Geometry check sheet. Reference: the model listing, model coordinates, mm. A direction names the side the tool comes from. Coordinates: 2 decimals unless noted, no trailing zeros. Write each loop counter-clockwise with the first axis right and the second up, starting at its lowest first coordinate (ties: lowest second). Pieces come first, ordered by that corner, then holes. Notation, with made-up numbers: (57, -2) - (70, -2) arc R16 ccw to (70, 15) - close; hole circle Ø6 at (60, -15). An arc over 180 degrees is marked (long way). Answer as a JSON object with one key per item and string values. Group by question number.
from build123d import *

# Parameters (mm, degrees)
F1_DEPTH = 15
F2_W     = 3.3
F2_H     = 1
F2_W_2   = 6.2084717173
F3_DEPTH = 13.301
F4_R     = 5


with BuildPart() as f1:
    # F0 (on Top) → F1 (new body)
    with BuildSketch(Plane.XY):
        with BuildLine():
            Line((6.65, 0), (1.65, 0))
            ThreePointArc((1.65, 0), (0, -1.65), (-1.65, 0))
            Line((-1.65, 0), (-6.65, 0))
            ThreePointArc((-6.65, 0), (0, -6.65), (6.65, 0))
        make_face()
        with BuildLine():
            ThreePointArc((-1.65, 0), (0, 1.65), (1.65, 0))
            Line((1.65, 0), (6.65, 0))
            ThreePointArc((6.65, 0), (0, 6.65), (-6.65, 0))
            Line((-6.65, 0), (-1.65, 0))
        make_face()
        with BuildLine():
            Line((6.65, -14), (6.65, 0))
            ThreePointArc((6.65, 0), (0, -6.65), (-6.65, 0))
            Line((-6.65, 0), (-6.65, -14))
            Line((-6.65, -14), (6.65, -14))
        make_face()
    extrude(amount=F1_DEPTH)

    # F2 (on face) → F3 (cut, through all)
    with BuildSketch(Plane.YZ.offset(6.65)):
        with BuildLine():
            ThreePointArc((-2.530230589, 7), (-2.5075645415, 7.2495434726), (-2.5, 7.5))
            ThreePointArc((-2.5, 7.5), (-2.5075645415, 7.7504565274), (-2.530230589, 8))
            Line((-2.530230589, 8), (-2.530230589, 7.5))
            Line((-2.530230589, 7.5), (-2.530230589, 7))
        make_face()
        with BuildLine():
            ThreePointArc((-2.530230589, 8), (-2.5075645415, 7.7504565274), (-2.5, 7.5))
            ThreePointArc((-2.5, 7.5), (-2.5075645415, 7.2495434726), (-2.530230589, 7))
            Line((-2.530230589, 7), (-1.65, 7))
            Line((-1.65, 7), (-1.65, 8))
            Line((-1.65, 8), (-2.530230589, 8))
        make_face()
        with BuildLine():
            Line((-2.530230589, 7.5), (-2.530230589, 8))
            ThreePointArc((-2.530230589, 8), (-6.9004565274, 11.6424354585), (-10.8, 7.5))
            Line((-10.8, 7.5), (-2.530230589, 7.5))
        make_face()
        with BuildLine():
            ThreePointArc((-10.8, 7.5), (-6.9004565274, 3.3575645415), (-2.530230589, 7))
            Line((-2.530230589, 7), (-2.530230589, 7.5))
            Line((-2.530230589, 7.5), (-10.8, 7.5))
        make_face()
        with Locations((0, 7.5)):
            Rectangle(F2_W, F2_H)
        with Locations((4.7542358587, 7.5)):
            Rectangle(F2_W_2, F2_H)
    extrude(amount=-F3_DEPTH, mode=Mode.SUBTRACT)

    # F4
    f4_edges = [f1.edges().sort_by_distance(p)[0] for p in [
        (0, -14, 15),
        (0, -14, 0),
    ]]
    fillet(f4_edges, radius=F4_R)


solid = f1.part
(1) Section check A-A (x = 0). Record the cut outline in (y, z).
(2) Section check B-B (z = 9.25). Record the cut outline in (x, y), and give its area (3 significant figures).
(3) Material ranges on L1, parallel to Y at x = 0, z = 11; L2, parallel to Z at x = -4.25, y = -0.5; L3, parallel to Y at x = 1.5, z = 8.75, recorded low to high. Write a range as [from, to].
(4) Draft check along Z on faces 1 (the face through (0, -3, 0)), 2 (the face through (-6.65, -4, 11)), 3 (the face through (0, -13, 13)), 4 (the face through (0, 2, 8)). Enter one of: +Z half, -Z half, draft (parallel to the pull), parting line (faces both ways), or undercut.
(5) Section check C-C (y = -6.65). Record the cut outline in (x, z), and give its area (3 significant figures).
(6) Section check D-D (z = 14). Record the cut outline in (x, y).
(7) Set-up check for faces 5 (the face through (0, 2, 7)), 6 (the face through (-1.574, 0.496, 3.451)): record each of +Z, -Z, +X, -X, +Y, -Y from which the full face is reachable in a straight line by a thin tool's end or side.
(8) Gauge pin test, flat end, axial feed: pin 1 (2.5 mm diameter, centred on x = 0, y = 0, fed in from -Z). Record the tip position at first contact, or that the pin passes through.
Conclusion:
{
 "1": {"outline": "(-14, 5) arc R5 ccw to (-9, 0) - (-1.65, 0) - (-1.65, 7) - (-2.53, 7) arc R4.15 cw (long way) to (-2.53, 8) - (-1.65, 8) - (-1.65, 15) - (-9, 15) arc R5 ccw to (-14, 10) - close; (1.65, 0) - (6.65, 0) - (6.65, 7) - (1.65, 7) - close; (1.65, 8) - (6.65, 8) - (6.65, 15) - (1.65, 15) - close"},
 "2": {"outline": "(-6.65, -14) - (6.65, -14) - (6.65, -10.41) - (-6.65, -10.41) - close; (-6.65, -2.89) - (6.65, -2.89) - (6.65, 0) arc R6.65 ccw to (-6.65, 0) - close; hole circle Ø3.3 at (0, 0)", "area": "147 mm^2"},
 "3": {"L1": "y = [-13.9, -8.88], [-4.42, -1.65], [1.65, 6.65]", "L2": "z = [0, 7], [8, 15]", "L3": "y = [-14, -10.61], [-2.69, -0.69], [0.69, 6.48]"},
 "4": {"face 1": "-Z half", "face 2": "draft", "face 3": "+Z half", "face 4": "undercut"},
 "5": {"outline": "(-6.65, 0) - (6.65, 0) - (6.65, 3.35) - (-6.65, 3.35) - close; (-6.65, 11.65) - (6.65, 11.65) - (6.65, 15) - (-6.65, 15) - close", "area": "89.1 mm^2"},
 "6": {"outline": "(-6.65, -12) - (6.65, -12) - (6.65, 0) arc R6.65 ccw to (-6.65, 0) - close; hole circle Ø3.3 at (0, 0)"},
 "7": {"face 5": "+X, -X, +Y", "face 6": "+Z, -Z"},
 "8": {"pin 1": "passes through"}
}
